Geometry: see drawing. Coordinates: mm, zero at the bounding-box minimum. A direction names the side the tool comes from. Round coordinates to 2 decimals unless told otherwise and drop trailing zeros. Write each loop counter-clockwise with the first axis right and the second up, starting at its lowest first coordinate (ties: lowest second). Pieces come first, ordered by that corner, then holes.
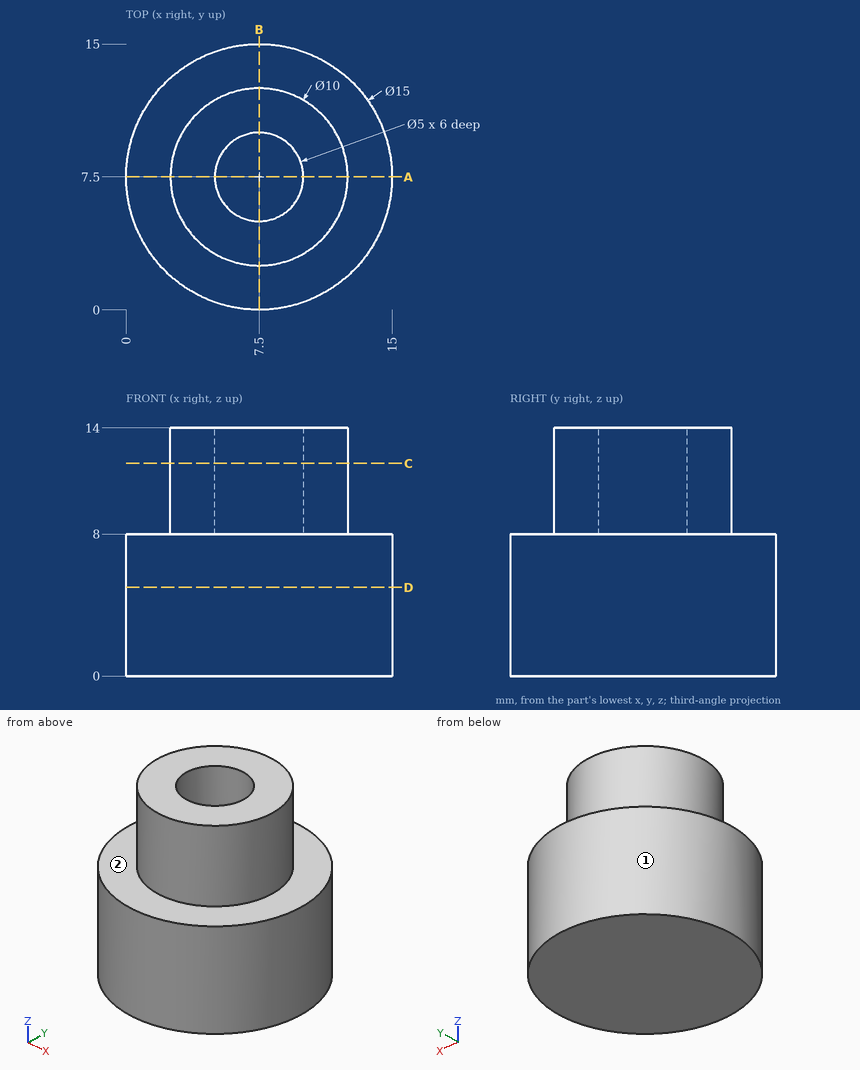
1) Material intervals for line 1 (Y direction, x = 7.5, z = 11.3); line 2 (Z direction, x = 11.75, y = 1.75); line 3 (Y direction, x = 7.75, z = 3.5), sorted ascending.
Taken from the geometry:
line 1: y = 2.5 to 5, 10 to 12.5
line 2: z = 0 to 8
line 3: y = 0 to 15
2) Section query A-A on y = 7.5. Return the cut outline in (x, z), then the cut area to 3 significant figures.
Taken from the geometry:
outline: (0, 0) - (15, 0) - (15, 8) - (12.5, 8) - (12.5, 14) - (10, 14) - (10, 8) - (5, 8) - (5, 14) - (2.5, 14) - (2.5, 8) - (0, 8) - close
area: 150 mm2
3) Reachability of the marked faces 1 and 2 from +Z, -Z, +X, -X, +Y, -Y: full face, straight path, thin tool, end or side. Return the list, or none.
Taken from the geometry:
face 1: +Z, -Z
face 2: +Z
4) Section query C-C on z = 12. Return the cut outline in (x, y), then the cut area to 3 significant figures.
Taken from the geometry:
outline: circle Ø10 at (7.5, 7.5); hole circle Ø5 at (7.5, 7.5)
area: 58.9 mm2
5) Contact query for flat-ended pins moving along their axis: P1, Ø6, axis at x = 11, z = 8.5, coming from the +Y side; P2, Ø5, axis at x = 6, y = 11, coming from the -Z side; P3, Ø1, axis at y = 10.5, z = 10.5, coming from the +X side; P4, Ø3, axis at x = 12.5, z = 10, coming from the +Y side. Output: stop coordinate, or through.
Taken from the geometry:
P1: stops at y = 14.98
P2: stops at z = 0
P3: stops at x = 11.83
P4: stops at y = 11.07
6) Section query D-D on z = 5. Return the cut outline in (x, y).
Taken from the geometry:
outline: circle Ø15 at (7.5, 7.5)
